from build123d import *

# Parameters (mm, degrees)
F1_DEPTH = 7.9375


# Not quite as in the source:
# - a length typed as a fraction of an inch, garbled in the dataset ("3 / 203.2 mm" for 3/8 in), is restored


with BuildPart() as f1:
    # F0 (on Top) → F1 (new body)
    with BuildSketch(Plane.XY):
        with BuildLine():
            ThreePointArc((-0.0986067535, 34.0497419238), (-4.0682176485, 31.9659465467), (-7.4162920937, 28.9842672646))
            ThreePointArc((-7.4162920937, 28.9842672646), (-8.8119305122, 25.5953281623), (-8.2258973271, 21.977417171))
            ThreePointArc((-8.2258973271, 21.977417171), (-9.7181261566, 18.698842434), (-9.2097157612, 15.1327075437))
            ThreePointArc((-9.2097157612, 15.1327075437), (-10.6205392688, 11.8246856933), (-10.2093555033, 8.2519613206))
            Line((-10.2093555033, 8.2519613206), (-12.369341217, 7.1464567445))
            Line((-12.369341217, 7.1464567445), (-12.369341217, 4.6386048198))
            Line((-12.369341217, 4.6386048198), (-12.369341217, 4.5682978211))
            ThreePointArc((-12.369341217, 4.5682978211), (-15.5930977879, 3.1185654947), (-17.7027139134, 0.2823972963))
            ThreePointArc((-17.7027139134, 0.2823972963), (-21.0452825194, -1.0603738309), (-23.1384971151, -3.9919692741))
            ThreePointArc((-23.1384971151, -3.9919692741), (-26.5647165348, -5.2934051439), (-28.80180468, -8.19653302))
            ThreePointArc((-28.80180468, -8.19653302), (-29.7673344436, -12.5572908836), (-29.5614041388, -17.0189104974))
            ThreePointArc((-29.5614041388, -17.0189104974), (-25.7783661022, -19.4669407743), (-21.4921734029, -20.8571857766))
            ThreePointArc((-21.4921734029, -20.8571857766), (-17.8594468391, -20.3713745504), (-15.0192606046, -18.054899429))
            ThreePointArc((-15.0192606046, -18.054899429), (-11.4338171794, -17.7079201351), (-8.5996589687, -15.484556372))
            ThreePointArc((-8.5996589687, -15.484556372), (-5.0294162563, -15.0523544446), (-2.1409380715, -12.9098966718))
            Line((-2.1409380715, -12.9098966718), (0, -14.2561570176))
            Line((0, -14.2561570176), (1.9696742658, -12.9098966718))
            ThreePointArc((1.9696742658, -12.9098966718), (4.9392756736, -15.0084468105), (8.560301624, -15.3410370587))
            ThreePointArc((8.560301624, -15.3410370587), (11.3944598347, -17.5644008218), (14.9799032599, -17.9113801157))
            ThreePointArc((14.9799032599, -17.9113801157), (17.8200894944, -20.2278552371), (21.4528160582, -20.7136664634))
            ThreePointArc((21.4528160582, -20.7136664634), (25.6558468929, -19.2922500665), (29.4813849032, -17.0447733253))
            ThreePointArc((29.4813849032, -17.0447733253), (29.5836204245, -12.511977875), (28.7624473353, -8.0530137067))
            ThreePointArc((28.7624473353, -8.0530137067), (26.5253591901, -5.1498858306), (23.0991397704, -3.8484499608))
            ThreePointArc((23.0991397704, -3.8484499608), (21.0059251747, -0.9168545176), (17.6633565687, 0.4259166096))
            ThreePointArc((17.6633565687, 0.4259166096), (15.4847616458, 3.3168082822), (12.1560195839, 4.739132713))
            Line((12.1560195839, 4.739132713), (12.1560195839, 7.1464567445))
            Line((12.1560195839, 7.1464567445), (9.9960338703, 8.2519613206))
            ThreePointArc((9.9960338703, 8.2519613206), (10.4072176357, 11.8246856933), (8.9963941282, 15.1327075437))
            ThreePointArc((8.9963941282, 15.1327075437), (9.5048045235, 18.698842434), (8.012575694, 21.977417171))
            ThreePointArc((8.012575694, 21.977417171), (8.5986088792, 25.5953281623), (7.2029704606, 28.9842672646))
            ThreePointArc((7.2029704606, 28.9842672646), (3.8655773676, 31.9687453881), (-0.0986067535, 34.0497419238))
        make_face()
    extrude(amount=F1_DEPTH)


solid = f1.part
CAD build for the part. Positions are in the model's coordinates, mm. A direction names the side the tool comes from. Coordinates: 2 decimals unless noted, no trailing zeros. Write each loop counter-clockwise with the first axis right and the second up, starting at its lowest first coordinate (ties: lowest second). Pieces come first, ordered by that corner, then holes. Notation, with made-up numbers: M 82.5,25 L 90.5,25 A30 ccw 90.5,60 Z; hole C -27,-17.5 d2. An arc over 180 degrees is marked long. Answer as a JSON object with one key per item and string values. Group by question number.
1) Saw through at B-B (x = -18.5). Write the cut outline in (y, z).
2) Pin check, flat tips, straight feed: pin 1 Ø1.9 at (y, z) = (6.5, 4.5) entering from +X; pin 2 Ø1.3 at (y, z) = (5.5, 4) entering from -X; pin 3 Ø1 at (x, z) = (-22, 4.5) entering from -Y. Stop position of each tip, or through.
3) Wall check: line 1 (X direction, y = 8, z = 2); line 2 (X direction, y = -14.5, z = 3.5); line 3 (X direction, y = -16, z = 2.75). Give the ranges that are in metal, low to high. Write a range as from..to.
4) Saw through at C-C (y = 3.5). Write the cut outline in (x, z), plus the area to 3 significant figures.
5) Tool access for faces 4 (the face through (-21.005, -1.029, 3.913)), 5 (the face through (0.971, -13.592, 3.913)), 6 (the face through (12.156, 6, 4)), 7 (the face through (-1, 1, 0)), 8 (the face through (-11.27, 7.71, 3.91)): list every direction of +Z, -Z, +X, -X, +Y, -Y with a clear straight run to the whole face (end or side of a thin tool).
6) Mould opens along X. For faces 1 (the face through (-10.613, 11.875, 3.913)), 2 (the face through (15.52, 3.29, 3.91)), 3 (the face through (-5.077, -15.071, 3.913)) say: +X half, -X half, draft (parallel to the pull), parting line (faces both ways), or undercut.
Values follow:
{
 "1": {"outline": "M -20.61,0 L 0.15,0 L 0.15,7.94 L -20.61,7.94 Z"},
 "2": {"pin 1": "stops at x = 12.16", "pin 2": "stops at x = -12.37", "pin 3": "stops at y = -20.86"},
 "3": {"line 1": "x = -10.7..10.49", "line 2": "x = -29.82..-3.93, 3.86..29.65", "line 3": "x = -29.71..-9.01, 9.1..29.59"},
 "4": {"outline": "M -15.07,0 L 15.24,0 L 15.24,7.94 L -15.07,7.94 Z", "area": "241 mm2"},
 "5": {"face 4": "+Z, -Z, -X, +Y", "face 5": "+Z, -Z, -Y", "face 6": "+Z, -Z, +X, +Y", "face 7": "-Z, +X, -X, +Y, -Y", "face 8": "+Z, -Z, -X"},
 "6": {"face 1": "-X half", "face 2": "+X half", "face 3": "undercut"}
}
